Model file for the job. Use its own axes, mm. Coordinates: 2 decimals unless noted, no trailing zeros. Put each result on its own line as item: value. Start each with the question number.
```python
from build123d import *

# Parameters (mm, degrees)
SKETCH1_R           = 1.5
BOSS_EXTRUDE1_DEPTH = 3
FILLET1_R           = 1
FILLET2_R           = 2


with BuildPart() as part:
    # Sketch1 → Boss-Extrude1 (new body)
    with BuildSketch(Plane.XY):
        with BuildLine():
            add(Edge.make_bspline(
                [(0, 0), (0.039034334, 61.604929497), (18.579234973, 120)],
                knots=[0, 0, 0, 1, 1, 1], degree=2))
            add(Edge.make_bspline(
                [(-18.032786885, 170), (-17.742349194, 156.285056374), (-6.538751715, 115.023114242), (17.720626912, 125.598656039), (18.579234973, 120)],
                knots=[0, 0, 0, 0, 0.447403359, 1, 1, 1, 1], degree=3))
            add(Edge.make_bspline(
                [(0, 0), (-19.47734459, 25.868323257), (-37.629056536, 125.986890488), (-18.032786885, 170)],
                knots=[0, 0, 0, 0, 1, 1, 1, 1], degree=3))
        make_face()
        with Locations((0.270016121, 65)):
            Circle(SKETCH1_R, mode=Mode.SUBTRACT)
        with Locations((0.270016121, 95)):
            Circle(SKETCH1_R, mode=Mode.SUBTRACT)
    extrude(amount=BOSS_EXTRUDE1_DEPTH)

    # Fillet1
    fillet1_edges = [part.edges().sort_by_distance(p)[0] for p in [
        (-18.032786885, 170, 1.5),
    ]]
    fillet(fillet1_edges, radius=FILLET1_R)

    # Fillet2
    fillet2_edges = [part.edges().sort_by_distance(p)[0] for p in [
        (0, 0, 1.5),
    ]]
    fillet(fillet2_edges, radius=FILLET2_R)


solid = part.part
```
Item 1: Flat gauge pin, fed straight in: pin 1 Ø1 at (y, z) = (49, 1.5) entering from -X. Where does the tip first touch, or does it go through?
Item 2: Pull direction Y, two halves, no side cores. Call faces 1 (the face through (-9, 87, 3)), 2 (the face through (0.075, 96.487, 1.479)): pulls with the +Y half, pulls with the -Y half, needs draft (parallel to the pull), parting line crosses it, or undercut.
Item 3: Slice it at A-A, the plane z = 0.5. Give the number of separate pieces and of enclosed holes in the cut face, plus the area to 3 significant figures.
Item 4: Wall check: line 1 along Y through (x, z) = (-1, 1.65); line 2 along X through (y, z) = (95, 0.7); line 3 along X through (y, z) = (130.5, 0.35). Give the ranges that are in metal, low to high.
Here are the results:
1. pin 1: stops at x = -18.55
2. face 1: needs draft
2. face 2: undercut
3. separate pieces: 1
3. enclosed holes: 2
3. area: 3,620 mm^2
4. line 1: y = 5 to 64.2, 65.8 to 94.2, 95.8 to 126.43
4. line 2: x = -25.49 to -1.23, 1.77 to 11.53
4. line 3: x = -26.12 to -5.79
